Work out the finished part from the listing and answer in its coordinate system (mm). A direction names the side the tool comes from. Coordinates: 2 decimals unless noted, no trailing zeros. Use a Markdown table: item, result.
from build123d import *

# Parameters (mm, degrees)
BOSS_EXTRUDE1_OUTLINE_R   = 2.5
BOSS_EXTRUDE1_OUTLINE_R_2 = 4.7
BOSS_EXTRUDE1_OUTLINE_R_3 = 5.8
BOSS_EXTRUDE1_OUTLINE_R_4 = 2
BOSS_EXTRUDE1_DEPTH       = 3
SKETCH3_R                 = 1.5
CUT_EXTRUDE1_DEPTH        = 2
SKETCH5_W                 = 62
SKETCH5_H                 = 18
SKETCH5_W_2               = 2
SKETCH5_H_2               = 2
CUT_EXTRUDE4_DEPTH        = 3
SKETCH6_R                 = 1.75
CUT_EXTRUDE5_DEPTH        = 3


# Read off the part's stored shape, not the designer's step: Boss-Extrude1
with BuildPart() as part:
    # Boss-Extrude1 outline → Boss-Extrude1 (new body)
    with BuildSketch(Plane(origin=(0, 0, 0), x_dir=(1, 0, 0), z_dir=(0, 1, 0))):
        with BuildLine():
            Line((-70, 78), (-119.123426788, 72.331912294))
            add(Edge.make_bspline(
                [(-119.123426788, 72.331912294), (-121.817313074, 72.000000019), (-122.273896674, 69.717527721)],
                knots=[0.016356922, 0.016356922, 0.016356922, 0.873306336, 0.873306336, 0.873306336], degree=2))
            Line((-122.273896674, 69.717527721), (-125, 47))
            add(Edge.make_bspline(
                [(-125, 47), (-140.310843166, 12.049240253), (-122.843906966, -52.183993971)],
                knots=[0, 0, 0, 0.96415889, 0.96415889, 0.96415889], degree=2))
            add(Edge.make_bspline(
                [(-122.843906966, -52.183993971), (-121.5, -57), (-118.282004102, -60.826813609)],
                knots=[0, 0, 0, 1, 1, 1], degree=2))
            add(Edge.make_bspline(
                [(-118.282004102, -60.826813609), (-103.606996493, -76.952025301), (-86.5, -72)],
                knots=[0.099631764, 0.099631764, 0.099631764, 1, 1, 1], degree=2))
            add(Edge.make_bspline(
                [(-86.5, -72), (0, -60), (86.5, -72)],
                knots=[0, 0, 0, 1, 1, 1], degree=2, weights=[1, 1.666666667, 1]))
            add(Edge.make_bspline(
                [(118.282004106, -60.826813605), (103.606996495, -76.952025301), (86.5, -72)],
                knots=[0.099631763, 0.099631763, 0.099631763, 1, 1, 1], degree=2))
            add(Edge.make_bspline(
                [(122.843906966, -52.183993971), (121.5, -57), (118.282004106, -60.826813605)],
                knots=[0, 0, 0, 1, 1, 1], degree=2))
            add(Edge.make_bspline(
                [(125, 47), (140.310843171, 12.049240242), (122.843906966, -52.183993971)],
                knots=[0, 0, 0, 0.96415889, 0.96415889, 0.96415889], degree=2))
            Line((125, 47), (122.273896674, 69.717527721))
            add(Edge.make_bspline(
                [(119.123426788, 72.331912294), (121.817313074, 72.000000019), (122.273896674, 69.717527721)],
                knots=[0.016356922, 0.016356922, 0.016356922, 0.873306336, 0.873306336, 0.873306336], degree=2))
            Line((119.123426788, 72.331912294), (70, 78))
            add(Edge.make_bspline(
                [(-70, 78), (0, 81), (70, 78)],
                knots=[0, 0, 0, 1, 1, 1], degree=2, weights=[1, 1.857142857, 1]))
        make_face()
        with Locations((-101.086868344, -59.874042945)):
            Circle(BOSS_EXTRUDE1_OUTLINE_R, mode=Mode.SUBTRACT)
        with Locations((-32.460031949, -46.153127094)):
            Circle(BOSS_EXTRUDE1_OUTLINE_R_2, mode=Mode.SUBTRACT)
        with Locations((-117.25, -21)):
            Circle(BOSS_EXTRUDE1_OUTLINE_R, mode=Mode.SUBTRACT)
        with BuildLine():
            Line((-70, -12), (-70, -29))
            add(Edge.make_bspline(
                [(-70, -29), (-70, -31.999987298), (-71.652526625, -34.50382822)],
                knots=[0, 0, 0, 1, 1, 1], degree=2))
            Line((-71.652526625, -34.50382822), (-85.673736688, -55.74808589))
            add(Edge.make_bspline(
                [(-85, -3), (-99, -3), (-112, 0), (-108, -8.5), (-105, -31), (-98, -49), (-94.5, -57), (-86.500030089, -57), (-85.673736688, -55.74808589)],
                knots=[0, 0, 0, 0, 0, 0, 0, 0, 0, 1, 1, 1, 1, 1, 1, 1, 1, 1], degree=8))
            Line((-85, -3), (-79, -3))
            ThreePointArc((-79, -3), (-72.636038969, -5.636038969), (-70, -12))
        make_face(mode=Mode.SUBTRACT)
        with Locations((-57.5, -23.153127094)):
            Circle(BOSS_EXTRUDE1_OUTLINE_R_3, mode=Mode.SUBTRACT)
        with Locations((0, -27.5)):
            Circle(BOSS_EXTRUDE1_OUTLINE_R_4, mode=Mode.SUBTRACT)
        with Locations((-23.815698604, -13.75)):
            Circle(BOSS_EXTRUDE1_OUTLINE_R_4, mode=Mode.SUBTRACT)
        with Locations((32.460031949, -46.153127094)):
            Circle(BOSS_EXTRUDE1_OUTLINE_R_2, mode=Mode.SUBTRACT)
        with Locations((101.086868344, -59.874042945)):
            Circle(BOSS_EXTRUDE1_OUTLINE_R, mode=Mode.SUBTRACT)
        with Locations((57.5, -23.153127094)):
            Circle(BOSS_EXTRUDE1_OUTLINE_R_3, mode=Mode.SUBTRACT)
        with Locations((23.815698604, -13.75)):
            Circle(BOSS_EXTRUDE1_OUTLINE_R_4, mode=Mode.SUBTRACT)
        with BuildLine():
            add(Edge.make_bspline(
                [(85, -3), (99, -3), (112, 0), (108, -8.5), (105, -31), (98, -49), (94.5, -57), (86.500030089, -57), (85.673736688, -55.74808589)],
                knots=[0, 0, 0, 0, 0, 0, 0, 0, 0, 1, 1, 1, 1, 1, 1, 1, 1, 1], degree=8))
            Line((85.673736688, -55.74808589), (71.652526625, -34.50382822))
            add(Edge.make_bspline(
                [(70, -29), (70, -31.999987298), (71.652526625, -34.50382822)],
                knots=[0, 0, 0, 1, 1, 1], degree=2))
            Line((70, -29), (70, -12))
            ThreePointArc((70, -12), (72.636038969, -5.636038969), (79, -3))
            Line((79, -3), (85, -3))
        make_face(mode=Mode.SUBTRACT)
        with Locations((117.25, -21)):
            Circle(BOSS_EXTRUDE1_OUTLINE_R, mode=Mode.SUBTRACT)
        with Locations((-88, 6)):
            Circle(BOSS_EXTRUDE1_OUTLINE_R, mode=Mode.SUBTRACT)
        with Locations((-117.3, 34.5)):
            Circle(BOSS_EXTRUDE1_OUTLINE_R, mode=Mode.SUBTRACT)
        with BuildLine():
            add(Edge.make_bspline(
                [(-105, 42), (-108, 15), (-92, 15), (-83.5, 15)],
                knots=[0, 0, 0, 0, 1, 1, 1, 1], degree=3))
            add(Edge.make_bspline(
                [(-85, 51), (-102.75, 51), (-105, 42)],
                knots=[0, 0, 0, 1, 1, 1], degree=2))
            ThreePointArc((-85, 51), (-74.393398282, 46.606601718), (-70, 36))
            Line((-70, 36), (-70, 24))
            ThreePointArc((-70, 24), (-72.636038969, 17.636038969), (-79, 15))
            Line((-79, 15), (-83.5, 15))
        make_face(mode=Mode.SUBTRACT)
        with Locations((-64.577794898, 6)):
            Circle(BOSS_EXTRUDE1_OUTLINE_R_3, mode=Mode.SUBTRACT)
        with Locations((-23.815698604, 13.75)):
            Circle(BOSS_EXTRUDE1_OUTLINE_R_4, mode=Mode.SUBTRACT)
        with Locations((-57.5, 29.977172881)):
            Circle(BOSS_EXTRUDE1_OUTLINE_R_3, mode=Mode.SUBTRACT)
        with Locations((0, 27.5)):
            Circle(BOSS_EXTRUDE1_OUTLINE_R_4, mode=Mode.SUBTRACT)
        with Locations((-111, 58)):
            Circle(BOSS_EXTRUDE1_OUTLINE_R_3, mode=Mode.SUBTRACT)
        with Locations((-86.612529585, 63.500116978)):
            Circle(BOSS_EXTRUDE1_OUTLINE_R_3, mode=Mode.SUBTRACT)
        with Locations((-63.376133298, 54.276783114)):
            Circle(BOSS_EXTRUDE1_OUTLINE_R_3, mode=Mode.SUBTRACT)
        with Locations((-31, 55.5)):
            Circle(BOSS_EXTRUDE1_OUTLINE_R_4, mode=Mode.SUBTRACT)
        with Locations((-31, 73.5)):
            Circle(BOSS_EXTRUDE1_OUTLINE_R_4, mode=Mode.SUBTRACT)
        with Locations((23.815698604, 13.75)):
            Circle(BOSS_EXTRUDE1_OUTLINE_R_4, mode=Mode.SUBTRACT)
        with Locations((64.577794898, 6)):
            Circle(BOSS_EXTRUDE1_OUTLINE_R_3, mode=Mode.SUBTRACT)
        with Locations((57.5, 29.977172881)):
            Circle(BOSS_EXTRUDE1_OUTLINE_R_3, mode=Mode.SUBTRACT)
        with Locations((88, 6)):
            Circle(BOSS_EXTRUDE1_OUTLINE_R, mode=Mode.SUBTRACT)
        with BuildLine():
            ThreePointArc((70, 36), (74.393398282, 46.606601718), (85, 51))
            add(Edge.make_bspline(
                [(85, 51), (102.75, 51), (105, 42)],
                knots=[0, 0, 0, 1, 1, 1], degree=2))
            add(Edge.make_bspline(
                [(105, 42), (108, 15), (92, 15), (83.5, 15)],
                knots=[0, 0, 0, 0, 1, 1, 1, 1], degree=3))
            Line((83.5, 15), (79, 15))
            ThreePointArc((79, 15), (72.636038969, 17.636038969), (70, 24))
            Line((70, 24), (70, 36))
        make_face(mode=Mode.SUBTRACT)
        with Locations((117.3, 34.5)):
            Circle(BOSS_EXTRUDE1_OUTLINE_R, mode=Mode.SUBTRACT)
        with Locations((31, 55.5)):
            Circle(BOSS_EXTRUDE1_OUTLINE_R_4, mode=Mode.SUBTRACT)
        with Locations((63.376133298, 54.276783114)):
            Circle(BOSS_EXTRUDE1_OUTLINE_R_3, mode=Mode.SUBTRACT)
        with Locations((31, 73.5)):
            Circle(BOSS_EXTRUDE1_OUTLINE_R_4, mode=Mode.SUBTRACT)
        with Locations((111, 58)):
            Circle(BOSS_EXTRUDE1_OUTLINE_R_3, mode=Mode.SUBTRACT)
        with Locations((86.612529585, 63.500116978)):
            Circle(BOSS_EXTRUDE1_OUTLINE_R_3, mode=Mode.SUBTRACT)
    extrude(amount=BOSS_EXTRUDE1_DEPTH)

    # Sketch3 → Cut-Extrude1 (cut)
    with BuildSketch(Plane.XZ):
        with Locations(Location((-25.085243816, 42.803127094, 0), (0, 0, 270))):
            Circle(SKETCH3_R)
        with Locations(Location((39.834820081, 42.803127094, 0), (0, 0, 270))):
            Circle(SKETCH3_R)
    extrude(amount=-CUT_EXTRUDE1_DEPTH, mode=Mode.SUBTRACT)

    # Sketch5 → Cut-Extrude4 (cut)
    with BuildSketch(Plane(origin=(0, 3, 0), x_dir=(1, 0, 0), z_dir=(0, 1, 0))):
        with Locations((0, 64.5)):
            Rectangle(SKETCH5_W, SKETCH5_H)
        with Locations((-32, 64.5)):
            Rectangle(SKETCH5_W_2, SKETCH5_H)
        with Locations((0, 74.5)):
            Rectangle(SKETCH5_W, SKETCH5_H_2)
        with Locations((0, 54.5)):
            Rectangle(SKETCH5_W, SKETCH5_H_2)
        with Locations((32, 64.5)):
            Rectangle(SKETCH5_W_2, SKETCH5_H)
    extrude(amount=-CUT_EXTRUDE4_DEPTH, mode=Mode.SUBTRACT)

    # Sketch6 → Cut-Extrude5 (cut)
    with BuildSketch(Plane(origin=(0, 3, 0), x_dir=(1, 0, 0), z_dir=(0, 1, 0))):
        with Locations(Location((-46.1, 72.949853444, 0), (0, 0, 270))):
            Circle(SKETCH6_R)
        with Locations(Location((-39.5, 47.95, 0), (0, 0, 270))):
            Circle(SKETCH6_R)
        with Locations(Location((39, 47.95, 0), (0, 0, 270))):
            Circle(SKETCH6_R)
        with Locations(Location((46.1, 72.949853444, 0), (0, 0, 270))):
            Circle(SKETCH6_R)
        with Locations(Location((-40.718373628, 73.152096314, 0), (0, 0, 270))):
            Circle(SKETCH6_R)
        with Locations(Location((40.718373628, 73.152096314, 0), (0, 0, 270))):
            Circle(SKETCH6_R)
    extrude(amount=-CUT_EXTRUDE5_DEPTH, mode=Mode.SUBTRACT)


solid = part.part
1. Flat-ended cylindrical pins translate along their axes: P1, Ø7, axis at x = 111, z = -58, coming from the -Y side; P2, Ø1.5, axis at y = 0.5, z = 7, coming from the +X side; P3, Ø2.5, axis at x = -25.09, z = 42.8, coming from the -Y side; P4, Ø0.9, axis at x = -81.5, y = 1, coming from the -Z side (3 decimals). Find the tip coordinate at first contact, or state that the pin passes through.
Answers below:
| item | result |
|---|---|
| P1 | through |
| P2 | x = 131.51 |
| P3 | y = 2 |
| P4 | z = -76.725 |
2. Section A-A on z = -6 is taken. Give the number of separate pieces and of enclosed holes in the cut face, then the cut area to 3 significant figures.
Answers below:
| item | result |
|---|---|
| separate pieces | 5 |
| enclosed holes | 0 |
| area | 693 mm² |
3. For a pull along Z with two mould halves and no side action, classify faces 1 (the face through (94.906, 1.479, -75.126)), 2 (the face through (-37.155, 1.479, 45.946)), 3 (the face through (72.706, 1.479, -17.566)), 4 (the face through (-2, 3, -3)) as +Z half, -Z half, draft (parallel to the pull), parting line (faces both ways), or undercut.
Answers below:
| item | result |
|---|---|
| face 1 | -Z half |
| face 2 | undercut |
| face 3 | undercut |
| face 4 | draft |
4. Find the intervals of material crossed by probe 1 along X at (y, z) = (1.05, -6); probe 2 along Z at (x, y) = (0, 1.95); probe 3 along X at (y, z) = (1.4, -24), in increasing order.
Answers below:
| item | result |
|---|---|
| probe 1 | -132.14 to -90.5, -85.5 to -70.38, -58.78 to 58.78, 70.38 to 85.5, 90.5 to 132.14 |
| probe 2 | -79.95 to -75.5, -53.5 to -29.5, -25.5 to 25.5, 29.5 to 64.5 |
| probe 3 | -131.16 to -103.16, -70 to 70, 103.16 to 131.16 |
5. For faces 5 (the face through (-2, 0, -3)), 6 (the face through (74.28, 1.48, -46.49)), determine the directions among +Z, -Z, +X, -X, +Y, -Y from which every point of the face is accessible in a straight line to the end or side of a thin tool.
Answers below:
| item | result |
|---|---|
| face 5 | +Z, -Z, +X, -X, -Y |
| face 6 | +Y, -Y |
